```python
from build123d import *

# Parameters (mm, degrees)
SKETCH_1_R          = 5
EXTRUDE_1_DEPTH     = 100
SKETCH_2_W          = 10
SKETCH_2_H          = 10
EXTRUDE_2_DEPTH     = 10
SKETCH_3_R          = 2.5
CUT_EXTRUDE_1_DEPTH = 101.623058987


with BuildPart() as part:
    # 草图1 → 凸台-拉伸1 (new body)
    with BuildSketch(Plane.XY):
        Circle(SKETCH_1_R)
    extrude(amount=EXTRUDE_1_DEPTH)

    # 草图2 → 凸台-拉伸2 (add)
    with BuildSketch(Plane(origin=(0, 0, 0), x_dir=(-1, 0, 0), z_dir=(0, 0, -1))):
        Rectangle(SKETCH_2_W, SKETCH_2_H)
    extrude(amount=EXTRUDE_2_DEPTH)

    # 草图3 → 切除-拉伸1 (cut, through all)
    with BuildSketch(Plane(origin=(5, 0, 0), x_dir=(0, 0, -1), z_dir=(1, 0, 0))):
        with Locations((5, 0)):
            Circle(SKETCH_3_R)
    extrude(amount=-CUT_EXTRUDE_1_DEPTH, mode=Mode.SUBTRACT)


solid = part.part
```
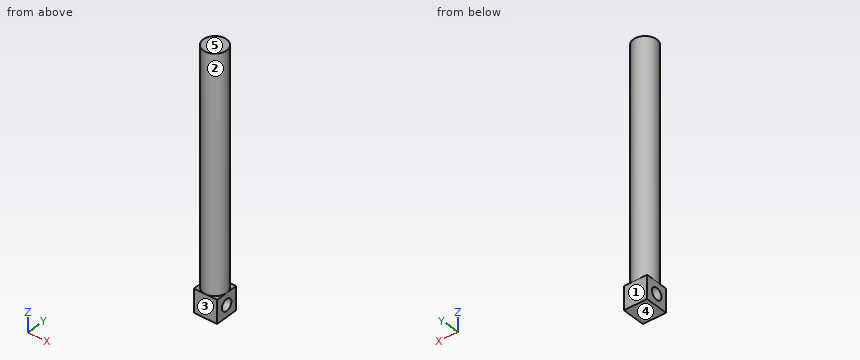
Check sheet for the modelled part. Datum: model origin and axes. Units: mm. Face numbers are marked on the shaded views. A direction names the side the tool comes from. Round coordinates to 2 decimals unless told otherwise and drop trailing zeros. Write each loop counter-clockwise with the first axis right and the second up, starting at its lowest first coordinate (ties: lowest second). Pieces come first, ordered by that corner, then holes. Notation, with made-up numbers: M 36.5,-28.5 L 64.5,-28.5 A10 ccw 64.5,-23.5 Z; hole C 11.25,46 d3. An arc over 180 degrees is marked long. Write item = value, one per line. Start each with the question number.
1. Section check B-B, the plane y = 1.5. Record the cut outline in (x, z).
2. Section check C-C, the plane x = 1. Record the cut outline in (y, z), then the cut area to 3 significant figures.
3. Scan lines: line 1 (Y direction, x = 2, z = -5); line 2 (Z direction, x = -3, y = 1); line 3 (X direction, y = 0.25, z = 83). Record each from-to range of solid material in increasing order. Write a range as [from, to].
4. Section check D-D, the plane z = 50.5. Record the cut outline in (x, y), then the cut area to 3 significant figures.
5. Section check A-A, the plane z = -5. Record the cut outline in (x, y), then the cut area to 3 significant figures.
6. Tool access check on the marked faces 1 and 2. Record the directions out of +Z, -Z, +X, -X, +Y, -Y that give a thin tool (end or side, any length) a straight path to the whole face; none if there is none.
7. Gauge pin test, flat ends, axial feed: pin 1 (1.5 mm diameter, centred on x = -1.5, z = 84, fed in from -Y); pin 2 (1 mm diameter, centred on x = -4, z = 18, fed in from +Y); pin 3 (3 mm diameter, centred on y = -3, z = 44, fed in from +X). Record the tip position at first contact, or that the pin passes through.
8. Release check for a two-part mould opening along Z. For the marked faces 3, 4 and 5 record: pulls with the +Z half, pulls with the -Z half, needs draft (parallel to the pull), parting line crosses it, or undercut.
Results found:
q1.outline = M -5,-10 L 5,-10 L 5,-7 L -5,-7 Z; M -5,-3 L 5,-3 L 5,0 L 4.77,0 L 4.77,100 L -4.77,100 L -4.77,0 L -5,0 Z
q2.outline = M -5,-10 L 5,-10 L 5,0 L 4.9,0 L 4.9,100 L -4.9,100 L -4.9,0 L -5,0 Z; hole C 0,-5 d5
q2.area = 1,060 mm^2
q3.line_1 = [-5, -2.5], [2.5, 5]
q3.line_2 = [-10, -7.29], [-2.71, 100]
q3.line_3 = [-4.99, 4.99]
q4.outline = C 0,0 d10
q4.area = 78.5 mm^2
q5.outline = M -5,-5 L 5,-5 L 5,-2.5 L -5,-2.5 Z; M -5,2.5 L 5,2.5 L 5,5 L -5,5 Z
q5.area = 50.0 mm^2
q6.face_1 = +Z, -Z, +X, -X, +Y
q6.face_2 = +Z
q7.pin_1 = -4.94
q7.pin_2 = 3.57
q7.pin_3 = 4.77
q8.face_3 = needs draft
q8.face_4 = pulls with the -Z half
q8.face_5 = pulls with the +Z half
